```python
from build123d import *

# Parameters (mm, degrees)
EXTRUDE_1_DEPTH     = 4
SKETCH_3_R          = 15
CUT_EXTRUDE_1_DEPTH = 5
SKETCH_4_R          = 2
CUT_EXTRUDE_2_DEPTH = 42.593268686
SKETCH_5_R          = 2
CUT_EXTRUDE_3_DEPTH = 49.95916666
SKETCH_6_R          = 13
CUT_EXTRUDE_4_DEPTH = 42.12177039


with BuildPart() as part:
    # 草图2 → 凸台-拉伸1 (new, symmetric)
    with BuildSketch(Plane.XY):
        Polygon((-25, 7), (-35, 7), (-35, 13), (-21, 13), (-21, 21), (21, 21), (21, 13), (35, 13), (35, 7), (25, 7), (25, 4), (21, 4), (21, -21), (-21, -21), (-21, 4), (-25, 4), align=None)
    extrude(amount=EXTRUDE_1_DEPTH, both=True)

    # 草图3 → 切除-拉伸1 (cut)
    with BuildSketch(Plane.XY.offset(4)):
        Circle(SKETCH_3_R)
    extrude(amount=-CUT_EXTRUDE_1_DEPTH, mode=Mode.SUBTRACT)

    # 草图4 → 切除-拉伸2 (cut, through all)
    with BuildSketch(Plane.XY.offset(4)):
        with Locations((-17.67766953, 17.67766953)):
            Circle(SKETCH_4_R)
        with Locations((17.67766953, 17.67766953)):
            Circle(SKETCH_4_R)
        with Locations((17.67766953, -17.67766953)):
            Circle(SKETCH_4_R)
        with Locations((-17.67766953, -17.67766953)):
            Circle(SKETCH_4_R)
    extrude(amount=-CUT_EXTRUDE_2_DEPTH, mode=Mode.SUBTRACT)

    # 草图5 → 切除-拉伸3 (cut, through all)
    with BuildSketch(Plane(origin=(0, 13, 0), x_dir=(1, 0, 0), z_dir=(0, 1, 0))):
        with Locations(Location((-30, 0, 0), (0, 0, 180))):
            Circle(SKETCH_5_R)
        with Locations(Location((30, 0, 0), (0, 0, 180))):
            Circle(SKETCH_5_R)
    extrude(amount=-CUT_EXTRUDE_3_DEPTH, mode=Mode.SUBTRACT)

    # 草图6 → 切除-拉伸4 (cut, through all)
    with BuildSketch(Plane.XY.offset(-1)):
        Circle(SKETCH_6_R)
    extrude(amount=-CUT_EXTRUDE_4_DEPTH, mode=Mode.SUBTRACT)


solid = part.part
```
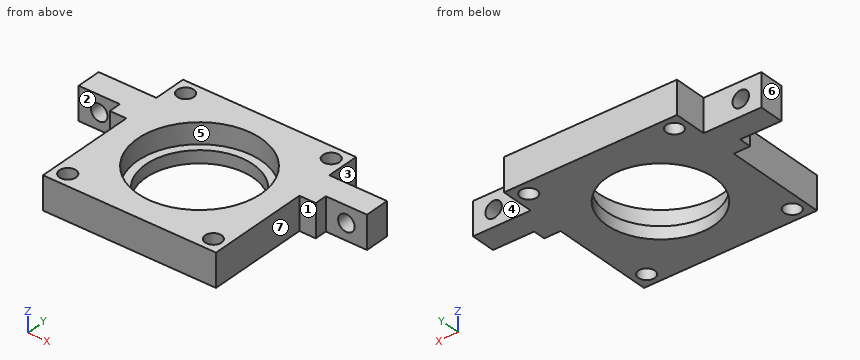
Model file for the job. Use its own axes, mm. Face numbers are marked on the shaded views. A direction names the side the tool comes from. Round coordinates to 2 decimals unless told otherwise and drop trailing zeros. Order: outer loops, then holes, each group sorted by start corner. A loop starts at its lowest first (then second) coordinate and runs counter-clockwise, first axis right, second up. Notation, with made-up numbers: (6, 35.25) -> (54, 35.25) arc R32 cw to (54, 69.25) -> close; hole circle Ø3 at (-12.5, 3.5). An arc over 180 degrees is marked (long way). Use one line per item in the form item = value.
Item 1: Tool access for the marked faces 1, 2 and 3: list every direction of +Z, -Z, +X, -X, +Y, -Y with a clear straight run to the whole face (end or side of a thin tool).
Returned:
face_1 = +Z, -Z, +X, -Y
face_2 = +Z, -Z, -X, -Y
face_3 = +Z, -Z, +X, +Y
Item 2: Flat gauge pins, fed straight in: pin 1 Ø4.5 at (x, z) = (-30, 0) entering from +Y; pin 2 Ø2.5 at (y, z) = (17.5, 1) entering from -X; pin 3 Ø4.5 at (x, z) = (30, 0) entering from -Y; pin 4 Ø3.5 at (x, y) = (17.68, -17.68) entering from -Z. Where does each tip first touch, or does it go through?
Returned:
pin_1 = 13
pin_2 = -21
pin_3 = 7
pin_4 = through
Item 3: Cut at B-B, the plane y = 11.5. Write the cut outline in (x, z), and give its area (3 significant figures).
Returned:
outline = (-35, -4) -> (-6.06, -4) -> (-6.06, -1) -> (-9.63, -1) -> (-9.63, 4) -> (-35, 4) -> close; (6.06, -4) -> (35, -4) -> (35, 4) -> (9.63, 4) -> (9.63, -1) -> (6.06, -1) -> close; hole circle Ø4 at (-30, 0); hole circle Ø4 at (30, 0)
area = 402 mm^2
Item 4: Pull direction X, two halves, no side cores. Call the marked faces 4, 5, 6 and 7: released by +X, released by -X, zero draft, split by the parting line, or undercut.
Returned:
face_4 = zero draft
face_5 = undercut
face_6 = released by -X
face_7 = released by +X
Item 5: Drill centre lines: line 1 (Y direction, x = 0, z = -2.2); line 2 (X direction, y = 16, z = 1.25); line 3 (Y direction, x = -31, z = 3.25). Where is each one in solid material? Low to high.
Returned:
line_1 = -21 to -13, 13 to 21
line_2 = -21 to -18.77, -16.59 to 16.59, 18.77 to 21
line_3 = 7 to 13
Item 6: Cut at A-A, the plane x = -30. Write the cut outline in (y, z), and give its area (3 significant figures).
Returned:
outline = (7, -4) -> (13, -4) -> (13, -2) -> (7, -2) -> close; (7, 2) -> (13, 2) -> (13, 4) -> (7, 4) -> close
area = 24.0 mm^2
Item 7: Cut at C-C, the plane z = 0. Give the number of separate pieces and of enclosed holes in the cut face, and give its area (3 significant figures).
Returned:
separate_pieces = 3
enclosed_holes = 5
area = 1,150 mm^2
Item 8: Cut at D-D, the plane x = 0. Write the cut outline in (y, z).
Returned:
outline = (-21, -4) -> (-13, -4) -> (-13, -1) -> (-15, -1) -> (-15, 4) -> (-21, 4) -> close; (13, -4) -> (21, -4) -> (21, 4) -> (15, 4) -> (15, -1) -> (13, -1) -> close
